Read the model definition and answer for the solid it produces. Units are mm, in the model's axes. A direction names the side the tool comes from. Give positions to 0.01 mm unless a question says otherwise; leave off trailing zeros. Order: outer loops, then holes, each group sorted by start corner. A loop starts at its lowest first (then second) coordinate and runs counter-clockwise, first axis right, second up. Notation, with made-up numbers: M 40,22.5 L 92,22.5 A5 cw 92,27.5 Z; hole C 4.5,-35 d7. An arc over 180 degrees is marked long. One line per item, written item: value. Start each with the question number.
from build123d import *

# Parameters (mm, degrees)
BOSS_EXTRUDE1_DEPTH     = 60
SKETCH2_R               = 2.5
CUT_EXTRUDE1_DEPTH      = 1
CUT_EXTRUDE1_DEPTH_BACK = 13
FILLET1_R               = 2


with BuildPart() as part:
    # Sketch1 → Boss-Extrude1 (new body)
    with BuildSketch(Plane(origin=(0, 0, 0), x_dir=(0, 0, -1), z_dir=(1, 0, 0))):
        Polygon((-50, 0), (0, 0), (0, -7), (7.5, -7), (7.5, -12), (-57.5, -12), (-57.5, -7), (-50, -7), align=None)
    extrude(amount=BOSS_EXTRUDE1_DEPTH)

    # Sketch2 → Cut-Extrude1 (cut, two sides)
    with BuildSketch(Plane(origin=(0, 0, 0), x_dir=(1, 0, 0), z_dir=(0, 1, 0))) as cut_extrude1_sk:
        with Locations((23, -10)):
            Circle(SKETCH2_R)
        with Locations((23, -40)):
            Circle(SKETCH2_R)
    extrude(amount=CUT_EXTRUDE1_DEPTH, mode=Mode.SUBTRACT)
    extrude(cut_extrude1_sk.sketch, amount=-CUT_EXTRUDE1_DEPTH_BACK, mode=Mode.SUBTRACT)

    # Fillet1
    fillet1_edges = [part.edges().sort_by_distance(p)[0] for p in [
        (20.5, 0, 10),
        (20.5, 0, 40),
    ]]
    fillet(fillet1_edges, radius=FILLET1_R)


solid = part.part
Q1. Find section D-D, the plane z = -2. Give the vertices of the cut face in (x, y).
Q2. A tool of negligible diameter and unlimited length cuts with its end or side. For faces 1 (the flat face through (30, -4, 50)), 2 (the flat face through (30, -7, -4)), 3 (the flat face through (30, -12, 25)), from which of +Z, -Z, +X, -X, +Y, -Y can it reach the whole face along a straight path? Write none if from no direction.
Q3. Determine the mould class of faces 4 (the flat face through (30, -10, 57.5)), 5 (the cylindrical face through (21, -6.9, 11.5)), 6 (the flat face through (30, -3, 0)) for opening direction Z: released by +Z, released by -Z, zero draft, split by the parting line, or undercut.
Q4. Consider probe 1 along Z at (x, y) = (23, -5); probe 2 along X at (y, z) = (-10.25, 10); probe 3 along Z at (x, y) = (17, -2.25). Determine where each line is inside the solid, lowest interval first.
Q5. Find section A-A, the plane x = 23. Give the vertices of the cut face in (y, z), then the cut area to 3 significant figures.
Q6. Find section B-B, the plane z = 10. Give the vertices of the cut face in (x, y), then the cut area to 3 significant figures.
Q7. Each of these flat-tipped pins is pushed along its axis until it touches: pin 1 (6 mm diameter, centred on x = 28.5, z = 55.5, fed in from +Y); pin 2 (2 mm diameter, centred on x = 15, y = -1.5, fed in from -Z). Where does it stop, or does it pass through?
Q8. Find section C-C, the plane x = 12. Give the vertices of the cut face in (y, z).
Evaluation:
1. outline: M 0,-12 L 60,-12 L 60,-7 L 0,-7 Z
2. face 1: +Z, +X, -X, +Y
2. face 2: -Z, +X, -X, +Y
2. face 3: +Z, -Z, +X, -X, -Y
3. face 4: released by +Z
3. face 5: undercut
3. face 6: released by -Z
4. probe 1: 0 to 7.5, 12.5 to 37.5, 42.5 to 50
4. probe 2: 0 to 20.5, 25.5 to 60
4. probe 3: 0 to 50
5. outline: M -12,-7.5 L -7,-7.5 L -7,0 L 0,0 L 0,5.5 A2 ccw -2,7.5 L -12,7.5 Z; M -12,12.5 L -2,12.5 A2 ccw 0,14.5 L 0,35.5 A2 ccw -2,37.5 L -12,37.5 Z; M -12,42.5 L -2,42.5 A2 ccw 0,44.5 L 0,50 L -7,50 L -7,57.5 L -12,57.5 Z
5. area: 552 mm2
6. outline: M 0,-12 L 20.5,-12 L 20.5,-2 A2 ccw 18.5,0 L 0,0 Z; M 25.5,-12 L 60,-12 L 60,0 L 27.5,0 A2 ccw 25.5,-2 Z
6. area: 658 mm2
7. pin 1: y = -7
7. pin 2: z = 0
8. outline: M -12,-7.5 L -7,-7.5 L -7,0 L 0,0 L 0,50 L -7,50 L -7,57.5 L -12,57.5 Z
